Work out the finished part from the listing and answer in its coordinate system (mm). A direction names the side the tool comes from. Round coordinates to 2 decimals unless told otherwise and drop trailing zeros. Loops run counter-clockwise (first coordinate to the right, second up) from the corner with the lowest first, then second, coordinate; pieces in that order, holes last. Notation, with made-up numbers: (4, 26.5) -> (28, 26.5) arc R24 ccw to (28, 53.5) -> close; hole circle Ø4 at (-8, 50.25). An arc over 180 degrees is marked (long way). Use CSV: the item, a comma, the result in double quotes. Start each with the question number.
from build123d import *

# Parameters (mm, degrees)
SKETCH2_R           = 11
SKETCH2_R_2         = 2.94
BOSS_EXTRUDE1_DEPTH = 9
SKETCH2_3_R         = 2.94
SKETCH2_3_R_2       = 1.55
BOSS_EXTRUDE2_DEPTH = 7
SKETCH2_4_R         = 2.94
SKETCH2_4_R_2       = 1.55
CUT_EXTRUDE1_DEPTH  = 3
SKETCH2_6_R         = 3.05
CUT_EXTRUDE2_DEPTH  = 8.6
SKETCH2_7_R         = 13
SKETCH2_7_R_2       = 11
BOSS_EXTRUDE3_DEPTH = 5.5


with BuildPart() as part:
    # Sketch2 → Boss-Extrude1 (new body)
    with BuildSketch(Plane(origin=(0, 0, 0), x_dir=(1, 0, 0), z_dir=(0, 1, 0))):
        with Locations(Location((0, 0, 0), (0, 0, 270))):
            Circle(SKETCH2_R)
        with Locations(Location((0, 0, 0), (0, 0, 270))):
            Circle(SKETCH2_R_2, mode=Mode.SUBTRACT)
    extrude(amount=BOSS_EXTRUDE1_DEPTH)

    # Sketch2<3> → Boss-Extrude2 (add)
    with BuildSketch(Plane(origin=(0, 0, 0), x_dir=(1, 0, 0), z_dir=(0, 1, 0))):
        with Locations(Location((0, 0, 0), (0, 0, 270))):
            Circle(SKETCH2_3_R)
        with Locations(Location((0, 0, 0), (0, 0, 270))):
            Circle(SKETCH2_3_R_2, mode=Mode.SUBTRACT)
    extrude(amount=BOSS_EXTRUDE2_DEPTH)

    # Sketch2<4> → Cut-Extrude1 (cut)
    with BuildSketch(Plane(origin=(0, 0, 0), x_dir=(1, 0, 0), z_dir=(0, 1, 0))):
        with Locations(Location((0, 0, 0), (0, 0, 270))):
            Circle(SKETCH2_4_R)
        with Locations(Location((0, 0, 0), (0, 0, 270))):
            Circle(SKETCH2_4_R_2, mode=Mode.SUBTRACT)
    extrude(amount=CUT_EXTRUDE1_DEPTH, mode=Mode.SUBTRACT)

    # Sketch2<6> → Cut-Extrude2 (cut)
    with BuildSketch(Plane(origin=(0, 0, 0), x_dir=(1, 0, 0), z_dir=(0, 1, 0))):
        with Locations(Location((5, 5, 0), (0, 0, 90))):
            Circle(SKETCH2_6_R)
        with Locations(Location((5, -5, 0), (0, 0, 90))):
            Circle(SKETCH2_6_R)
        with Locations(Location((-5, -5, 0), (0, 0, 90))):
            Circle(SKETCH2_6_R)
        with Locations(Location((-5, 5, 0), (0, 0, 90))):
            Circle(SKETCH2_6_R)
    extrude(amount=CUT_EXTRUDE2_DEPTH, mode=Mode.SUBTRACT)

    # Sketch2<7> → Boss-Extrude3 (add)
    with BuildSketch(Plane(origin=(0, 0, 0), x_dir=(1, 0, 0), z_dir=(0, 1, 0))):
        with Locations(Location((0, 0, 0), (0, 0, 270))):
            Circle(SKETCH2_7_R)
        with Locations(Location((0, 0, 0), (0, 0, 270))):
            Circle(SKETCH2_7_R_2, mode=Mode.SUBTRACT)
    extrude(amount=BOSS_EXTRUDE3_DEPTH)


solid = part.part
Q1. Which of the six approach directions +Z, -Z, +X, -X, +Y, -Y give full straight-line access (tool end or side, diameter ignored) to faces 1 (the cylindrical face through (7.706, 4.24, -6.407)), 2 (the cylindrical face through (0.9, 8, 2.8)), 3 (the cylindrical face through (-7.91, 2.712, -10.316))?
Q2. For a pull along X with two mould halves and no side action, classify faces 4 (the flat face through (-1.3, 3, 1.3)), 5 (the cylindrical face through (-10.74, 7.23, -2.38)), 6 (the flat face through (3, 5.5, -11)), 7 (the cylindrical face through (0.9, 1.5, 2.8)) as pulls with the +X half, pulls with the -X half, needs draft (parallel to the pull), parting line crosses it, or undercut.
Q3. Section D-D, the plane x = 2.5 is taken. Write down the section's boundary in (y, z), and give its area (3 significant figures).
Q4. Section A-A, the plane z = 0 is taken. Write down the section's boundary in (x, y).
Q5. Section C-C, the plane x = -1 is taken. Write down the section's boundary in (y, z), and give its area (3 significant figures).
Q6. Straight lines are drawn through the part: line 1 (X direction, y = 2.5, z = -4); line 2 (Z direction, x = -7.25, y = 4.25); line 3 (X direction, y = 4.05, z = 0). For each, find the intervals that lie inside material, in ascending order. Write a range as from..to.
Q7. Each of these flat-tipped pins is pushed along its axis until it touches: pin 1 (3.5 mm diameter, centred on x = 0, z = 0, fed in from +Y); pin 2 (3.5 mm diameter, centred on x = -5, z = -5, fed in from -Y); pin 3 (6.5 mm diameter, centred on x = -0.5, z = 1.5, fed in from -Y); pin 4 (3.5 mm diameter, centred on x = 0, z = 0, fed in from -Y). Where does it stop, or does it pass through?
Q8. Section B-B, the plane y = 6.25 is taken. Write down the section's boundary in (x, z), and give its area (3 significant figures).
Report:
1,face 1,"-Y"
1,face 2,"+Y"
1,face 3,"+Y, -Y"
2,face 4,"undercut"
2,face 5,"parting line crosses it"
2,face 6,"needs draft"
2,face 7,"undercut"
3,outline,"(0, -12.76) -> (5.5, -12.76) -> (5.5, -10.71) -> (9, -10.71) -> (9, -1.55) -> (7, -1.55) -> (7, 1.55) -> (9, 1.55) -> (9, 10.71) -> (5.5, 10.71) -> (5.5, 12.76) -> (0, 12.76) -> (0, 6.75) -> (8.6, 6.75) -> (8.6, 3.25) -> (0, 3.25) -> (0, 1.55) -> (3, 1.55) -> (3, -1.55) -> (0, -1.55) -> (0, -3.25) -> (8.6, -3.25) -> (8.6, -6.75) -> (0, -6.75) -> close"
3,area,"140 mm²"
4,outline,"(-13, 0) -> (-2.94, 0) -> (-2.94, 3) -> (-1.55, 3) -> (-1.55, 7) -> (-2.94, 7) -> (-2.94, 9) -> (-11, 9) -> (-11, 5.5) -> (-13, 5.5) -> close; (1.55, 3) -> (2.94, 3) -> (2.94, 0) -> (13, 0) -> (13, 5.5) -> (11, 5.5) -> (11, 9) -> (2.94, 9) -> (2.94, 7) -> (1.55, 7) -> close"
5,outline,"(0, -12.96) -> (5.5, -12.96) -> (5.5, -10.95) -> (9, -10.95) -> (9, -2.76) -> (7, -2.76) -> (7, -1.18) -> (3, -1.18) -> (3, -2.76) -> (0, -2.76) -> close; (0, 2.76) -> (3, 2.76) -> (3, 1.18) -> (7, 1.18) -> (7, 2.76) -> (9, 2.76) -> (9, 10.95) -> (5.5, 10.95) -> (5.5, 12.96) -> (0, 12.96) -> close"
5,area,"182 mm²"
6,line 1,"x = -12.37..-7.88, -2.12..2.12, 7.88..12.37"
6,line 2,"z = -10.79..-7.06, -2.94..2.94, 7.06..10.79"
6,line 3,"x = -13..-1.55, 1.55..13"
7,pin 1,"stops at y = 7"
7,pin 2,"stops at y = 8.6"
7,pin 3,"stops at y = 0"
7,pin 4,"stops at y = 3"
8,outline,"circle Ø22 at (0, 0); hole circle Ø6.1 at (-5, -5); hole circle Ø6.1 at (-5, 5); hole circle Ø3.1 at (0, 0); hole circle Ø6.1 at (5, -5); hole circle Ø6.1 at (5, 5)"
8,area,"256 mm²"
